from build123d import *

# Parameters (mm, degrees)
SKETCH1_R           = 8
SKETCH1_R_2         = 7
BOSS_EXTRUDE1_DEPTH = 1
FILLET1_R           = 0.25
FILLET2_R           = 0.25
FILLET3_R           = 0.25
FILLET4_R           = 0.25


with BuildPart() as part:
    # Sketch1 → Boss-Extrude1 (new body)
    with BuildSketch(Plane.XY):
        Circle(SKETCH1_R)
        Circle(SKETCH1_R_2, mode=Mode.SUBTRACT)
    extrude(amount=BOSS_EXTRUDE1_DEPTH)

    # Fillet1
    fillet1_edges = [part.edges().sort_by_distance(p)[0] for p in [
        (-8, 0, 1),
    ]]
    fillet(fillet1_edges, radius=FILLET1_R)

    # Fillet2
    fillet2_edges = [part.edges().sort_by_distance(p)[0] for p in [
        (-7, 0, 1),
    ]]
    fillet(fillet2_edges, radius=FILLET2_R)

    # Fillet3
    fillet3_edges = [part.edges().sort_by_distance(p)[0] for p in [
        (-8, 0, 0),
    ]]
    fillet(fillet3_edges, radius=FILLET3_R)

    # Fillet4
    fillet4_edges = [part.edges().sort_by_distance(p)[0] for p in [
        (-7, 0, 0),
    ]]
    fillet(fillet4_edges, radius=FILLET4_R)


solid = part.part
Can you work these out from the model? Positions are in its coordinate system, mm. Round coordinates to 2 decimals unless told otherwise and drop trailing zeros. Loops run counter-clockwise (first coordinate to the right, second up) from the corner with the lowest first, then second, coordinate; pieces in that order, holes last. Notation, with made-up numbers: (46, 54.5) - (70, 54.5) arc R15 cw to (70, 72.5) - close; hole circle Ø3 at (-24.5, 42). An arc over 180 degrees is marked (long way). Use CSV: the item, a comma, the result in double quotes. Start each with the question number.
1) If we section it at A-A on x = 0: Write out the boundary of the cut face in (y, z).
2) If we section it at C-C on z = 0.55: Write out the boundary of the cut face in (x, y).
3) We'd pull the mould along X, two halves only. Please class faces 1 (the cylindrical face through (6.466, -2.681, 0.496)), 2 (the cylindrical face through (-1.73, -7.81, 0.5)), 3 (the flat face through (2.8, -6.9, 0)): released by +X, released by -X, zero draft, split by the parting line, or undercut.
4) Please list where these lines run through material, in increasing order: probe 1 along Y at (x, z) = (0, 0.4); probe 2 along X at (y, z) = (4, 0.55); probe 3 along Y at (x, z) = (-1, 0.8). Write a range as [from, to].
Geometry results:
1,outline,"(-8, 0.25) arc R0.25 ccw to (-7.75, 0) - (-7.25, 0) arc R0.25 ccw to (-7, 0.25) - (-7, 0.75) arc R0.25 ccw to (-7.25, 1) - (-7.75, 1) arc R0.25 ccw to (-8, 0.75) - close; (7, 0.25) arc R0.25 ccw to (7.25, 0) - (7.75, 0) arc R0.25 ccw to (8, 0.25) - (8, 0.75) arc R0.25 ccw to (7.75, 1) - (7.25, 1) arc R0.25 ccw to (7, 0.75) - close"
2,outline,"circle Ø16 at (0, 0); hole circle Ø14 at (0, 0)"
3,face 1,"undercut"
3,face 2,"split by the parting line"
3,face 3,"zero draft"
4,probe 1,"y = [-8, -7], [7, 8]"
4,probe 2,"x = [-6.93, -5.74], [5.74, 6.93]"
4,probe 3,"y = [-7.93, -6.93], [6.93, 7.93]"
